```python
from build123d import *

# Parameters (mm, degrees)
F1_R        = 1.6
F2_DEPTH    = 8
F3_R        = 2.85
F4_DEPTH    = 3
F6_DEPTH    = 2.5
F7_D        = 3.2
F8_T1_DEPTH = 23


# Not quite as in the source:
# - a fillet or chamfer that OpenCascade refuses, or shapes differently, is made with other operations: its cross-section is extruded or revolved along the edge and cut away or added


with BuildPart() as f2:
    # F1 (on Top) → F2 (new body)
    with BuildSketch(Plane.XY):
        Polygon((45.5, -7), (45.5, 0), (45.5, 4), (-14.5, 4), (-14.5, 0), (-14.5, -0.2), (-14.5, -7), (-9.5, -7), (40.5, -7), align=None)
        Circle(F1_R, mode=Mode.SUBTRACT)
        with Locations((31, 0)):
            Circle(F1_R, mode=Mode.SUBTRACT)
    extrude(amount=F2_DEPTH)

    # F3 (on face) → F4 (cut)
    with BuildSketch(Plane.XY.offset(8)):
        Circle(F3_R)
        with Locations((31, 0)):
            Circle(F3_R)
    extrude(amount=-F4_DEPTH, mode=Mode.SUBTRACT)

    # F5 (on face) → F6 (cut)
    with BuildSketch(Plane.XZ.offset(7)):
        Polygon((-7.9122867597, 6.75), (-11.0877132403, 6.75), (-12.6754264805, 4), (-11.0877132403, 1.25), (-7.9122867597, 1.25), (-6.3245735195, 4), align=None)
        Polygon((11.0877132403, 6.75), (7.9122867597, 6.75), (6.3245735195, 4), (7.9122867597, 1.25), (11.0877132403, 1.25), (12.6754264805, 4), align=None)
    extrude(amount=-F6_DEPTH, mode=Mode.SUBTRACT)

    # F7 (through all)
    with Locations(Plane.XZ.offset(7)):
        with Locations((-9.5, 4), (9.5, 4)):
            Hole(F7_D / 2)

    # F8: fillet of radius 3 on 4 edges, made by hand

    # F8_s2 → F8_t1 (cut)
    with BuildSketch(Plane.XY.offset(-7.5)):
        with BuildLine():
            ThreePointArc((-11.5, 4), (-13.6213203436, 3.1213203436), (-14.5, 1))
            Line((-14.5, 1), (-14.5, 4))
            Line((-14.5, 4), (-11.5, 4))
        make_face()
        with BuildLine():
            ThreePointArc((45.5, -4), (44.6213203436, -6.1213203436), (42.5, -7))
            Line((42.5, -7), (45.5, -7))
            Line((45.5, -7), (45.5, -4))
        make_face()
        with BuildLine():
            ThreePointArc((45.5, 1), (44.6213203436, 3.1213203436), (42.5, 4))
            Line((42.5, 4), (45.5, 4))
            Line((45.5, 4), (45.5, 1))
        make_face()
        with BuildLine():
            ThreePointArc((-11.5, -7), (-13.6213203436, -6.1213203436), (-14.5, -4))
            Line((-14.5, -4), (-14.5, -7))
            Line((-14.5, -7), (-11.5, -7))
        make_face()
    extrude(amount=F8_T1_DEPTH, mode=Mode.SUBTRACT)


solid = f2.part
```
Can you work these out from the model? Positions are in its coordinate system, mm. A direction names the side the tool comes from. Round coordinates to 2 decimals unless told otherwise and drop trailing zeros. Order: outer loops, then holes, each group sorted by start corner. A loop starts at its lowest first (then second) coordinate and runs counter-clockwise, first axis right, second up. Notation, with made-up numbers: (38.5, -24.5) -> (43.5, -24.5) arc R18 cw to (43.5, -18.5) -> close; hole circle Ø3 at (64.5, -29.5). An arc over 180 degrees is marked (long way). Return JSON: item names as keys, results as strings. Group by question number.
1. Which directions (+Z, -Z, +X, -X, +Y, -Y) give clear straight access to the entire face, cutting with the end or side of a thin tool? Please do faces 1 (the face through (11.1, -0.19, 4.07)), 2 (the face through (-9, -6, 6.75)), 3 (the face through (-2.262, -1.734, 6.521)).
2. Will these pins go through, and if not, where does the flat tip stop? pin 1 (5 mm diameter, centred on x = 31, y = 0, fed in from +Z); pin 2 (1.6 mm diameter, centred on x = 9, z = 3.5, fed in from -Y); pin 3 (3.5 mm diameter, centred on x = 9.5, z = 4, fed in from -Y).
3. If we section it at A-A, the plane y = 0: Write out the boundary of the cut face in (x, z), then the cut area to 3 significant figures.
4. We'd pull the mould along X, two halves only. Please class faces 4 (the face through (-7.11, -5.77, 5.36)), 5 (the face through (-13.6, 3.14, 3.94)), 6 (the face through (44.64, 3.1, 3.94)), 7 (the face through (9, -6, 1.25)): released by +X, released by -X, zero draft, split by the parting line, or undercut.
5. I need wall thicknesses on line 1 (X direction, y = 0, z = 1.5); line 2 (Z direction, x = 9.5, y = -2); line 3 (Y direction, x = 31, z = 6.25). Which ranges of each line are inside material? Lowest first, please. Write a range as [from, to].
6. If we section it at B-B, the plane x = 9.5: Write out the boundary of the cut face in (y, z), then the cut area to 4 significant figures.
7. If we section it at C-C, the plane x = 0: Write out the boundary of the cut face in (y, z), then the cut area to 3 significant figures.
Output values:
{
 "1": {"face 1": "+Y, -Y", "face 2": "-Y", "face 3": "+Z"},
 "2": {"pin 1": "z = 5", "pin 2": "through", "pin 3": "y = -4.5"},
 "3": {"outline": "(-14.5, 0) -> (-1.6, 0) -> (-1.6, 5) -> (-2.85, 5) -> (-2.85, 8) -> (-14.5, 8) -> close; (1.6, 0) -> (29.4, 0) -> (29.4, 5) -> (28.15, 5) -> (28.15, 8) -> (2.85, 8) -> (2.85, 5) -> (1.6, 5) -> close; (32.6, 0) -> (45.5, 0) -> (45.5, 8) -> (33.85, 8) -> (33.85, 5) -> (32.6, 5) -> close; hole circle Ø3.2 at (-9.5, 4); hole circle Ø3.2 at (9.5, 4)", "area": "398 mm²"},
 "4": {"face 4": "undercut", "face 5": "released by -X", "face 6": "released by +X", "face 7": "undercut"},
 "5": {"line 1": "[-14.5, -1.6], [1.6, 29.4], [32.6, 45.5]", "line 2": "[0, 2.4], [5.6, 8]", "line 3": "[-7, -2.85], [2.85, 4]"},
 "6": {"outline": "(-7, 0) -> (4, 0) -> (4, 2.4) -> (-4.5, 2.4) -> (-4.5, 1.25) -> (-7, 1.25) -> close; (-7, 6.75) -> (-4.5, 6.75) -> (-4.5, 5.6) -> (4, 5.6) -> (4, 8) -> (-7, 8) -> close", "area": "47.05 mm²"},
 "7": {"outline": "(-7, 0) -> (-1.6, 0) -> (-1.6, 5) -> (-2.85, 5) -> (-2.85, 8) -> (-7, 8) -> close; (1.6, 0) -> (4, 0) -> (4, 8) -> (2.85, 8) -> (2.85, 5) -> (1.6, 5) -> close", "area": "54.9 mm²"}
}
